The listing builds one solid part. Answer for the finished solid, in the listing's coordinates (mm). A direction names the side the tool comes from. Round coordinates to 2 decimals unless told otherwise and drop trailing zeros. Order: outer loops, then holes, each group sorted by start corner. A loop starts at its lowest first (then second) coordinate and runs counter-clockwise, first axis right, second up. Notation, with made-up numbers: (86, 15.5) - (124, 15.5) arc R21 ccw to (124, 37.5) - close; hole circle Ø11 at (-19.75, -37). An arc over 180 degrees is marked (long way). Use CSV: the item, a comma, the result in double quotes. Start each with the question number.
Item 1: Find section D-D, the plane y = 0.85. Give the vertices of the cut face in (x, z) (3 decimals).
Item 2: For faces 1 (the cylindrical face through (0.109, 1.048, -2.873)), 2 (the flat face through (-1.85, 1.08, 6.92)), 3 (the flat face through (-1.832, 3.202, 6.922)), determine the directions among +Z, -Z, +X, -X, +Y, -Y from which every point of the face is accessible in a straight line to the end or side of a thin tool.
Item 3: Find section B-B, the plane z = 9.75. Give the vertices of the cut face in (x, y) (3 decimals).
Item 4: Flat-ended cylindrical pins translate along their axes: P1, Ø1.2, axis at x = -0.5, z = 6.5, coming from the +Y side; P2, Ø1, axis at x = 2, z = 7.5, coming from the -Y side. Find the tip coordinate at first contact, or state that the pin passes through.
Item 5: Straight lines are drawn through the part: line 1 along Y through (x, z) = (0, 5.25); line 2 along X through (y, z) = (1.25, 0) (3 decimals); line 3 along Z through (x, y) = (1, 3.2). For each, find the intervals that lie inside material, in ascending order. Write a range as [from, to].
Item 6: Determine the mould class of faces 4 (the cylindrical face through (-0.608, 3.078, 7.06)), 5 (the flat face through (0, 0, 6)), 6 (the flat face through (1.85, 3.17, 6.92)) for opening direction X: +X half, -X half, draft (parallel to the pull), parting line (faces both ways), or undercut.
Item 7: Find section C-C, the plane z = 0. Give the vertices of the cut face in (x, y) (3 decimals), plus the area to 3 significant figures.
```python
from build123d import *

# Parameters (mm, degrees)
BOSS_EXTRUDE1_DEPTH       = 12.5
F_4_40_TAPPED_HOLE1_D     = 2.2606
F_4_40_TAPPED_HOLE1_DEPTH = 12
F_4_40_TAPPED_HOLE1_TIP   = 0.679152758
CHAMFER1_SIZE             = 0.375


with BuildPart() as part:
    # Sketch1 → Revolve1 (revolve)
    with BuildSketch(Plane.XY):
        with BuildLine():
            Line((2.875, 2.125), (2.875, 0))
            Line((2.875, 0), (0, 0))
            Line((0, 0), (0, 5))
            ThreePointArc((0, 5), (2.032931996, 4.157931996), (2.875, 2.125))
        make_face()
    revolve(axis=Axis((0, 0, 0), (0, 1, 0)))

    # Sketch2 → Boss-Extrude1 (add)
    with BuildSketch(Plane.XY):
        Polygon((-1.226869322, 0), (1.226869322, 0), (2.453738644, 2.125), (1.226869322, 4.25), (-1.226869322, 4.25), (-2.453738644, 2.125), align=None)
    extrude(amount=BOSS_EXTRUDE1_DEPTH)

    # #4-40 Tapped Hole1
    with Locations(Plane.XY.offset(12.5)):
        with Locations((0, 2.125)):
            Hole(F_4_40_TAPPED_HOLE1_D / 2, depth=F_4_40_TAPPED_HOLE1_DEPTH)
            with Locations((0, 0, -(F_4_40_TAPPED_HOLE1_DEPTH + F_4_40_TAPPED_HOLE1_TIP / 2))):  # 118° drill point
                Cone(0, F_4_40_TAPPED_HOLE1_D / 2, F_4_40_TAPPED_HOLE1_TIP, mode=Mode.SUBTRACT)

    # Sketch5 → Cut-Revolve1 (revolve, cut)
    with BuildSketch(Plane(origin=(0, 0, 0), x_dir=(0, 0, -1), z_dir=(1, 0, 0))):
        with BuildLine():
            Line((2.1, 2.125), (2.1, 0))
            Line((2.1, 0), (0, 0))
            Line((0, 0), (0, 4.225))
            ThreePointArc((0, 4.225), (1.48492424, 3.60992424), (2.1, 2.125))
        make_face()
    revolve(axis=Axis((0, 0, 0), (0, 1, 0)), mode=Mode.SUBTRACT)

    # Chamfer1
    chamfer1_edges = [part.edges().sort_by_distance(p)[0] for p in [
        (0, 0, 2.1),
    ]]
    chamfer(chamfer1_edges, length=CHAMFER1_SIZE)


solid = part.part
```
Worked out:
1,outline,"(-1.718, 2.306) arc R2.875 ccw (long way) to (1.718, 2.306) - (1.718, 12.5) - (-1.718, 12.5) - close; hole circle Ø4.2 at (0, 0)"
2,face 1,"-Y"
2,face 2,"+Z, -X, -Y"
2,face 3,"+Z, -X, +Y"
3,outline,"(-2.454, 2.125) - (-1.227, 0) - (1.227, 0) - (2.454, 2.125) - (1.227, 4.25) - (-1.227, 4.25) - close; hole circle Ø2.261 at (0, 2.125)"
4,P1,"stops at y = 4.25"
4,P2,"stops at y = 0.47"
5,line 1,"y = [0, 0.99], [3.26, 4.25]"
5,line 2,"x = [-2.875, -2.1], [2.1, 2.875]"
5,line 3,"z = [-2.47, -1.5], [1.5, 12.5]"
6,face 4,"undercut"
6,face 5,"draft"
6,face 6,"+X half"
7,outline,"(-2.875, 0) - (-2.475, 0) - (-2.1, 0.375) - (-2.1, 2.125) arc R2.1 cw to (2.1, 2.125) - (2.1, 0.375) - (2.475, 0) - (2.875, 0) - (2.875, 2.125) arc R2.875 ccw to (-2.875, 2.125) - close"
7,area,"9.21 mm²"
